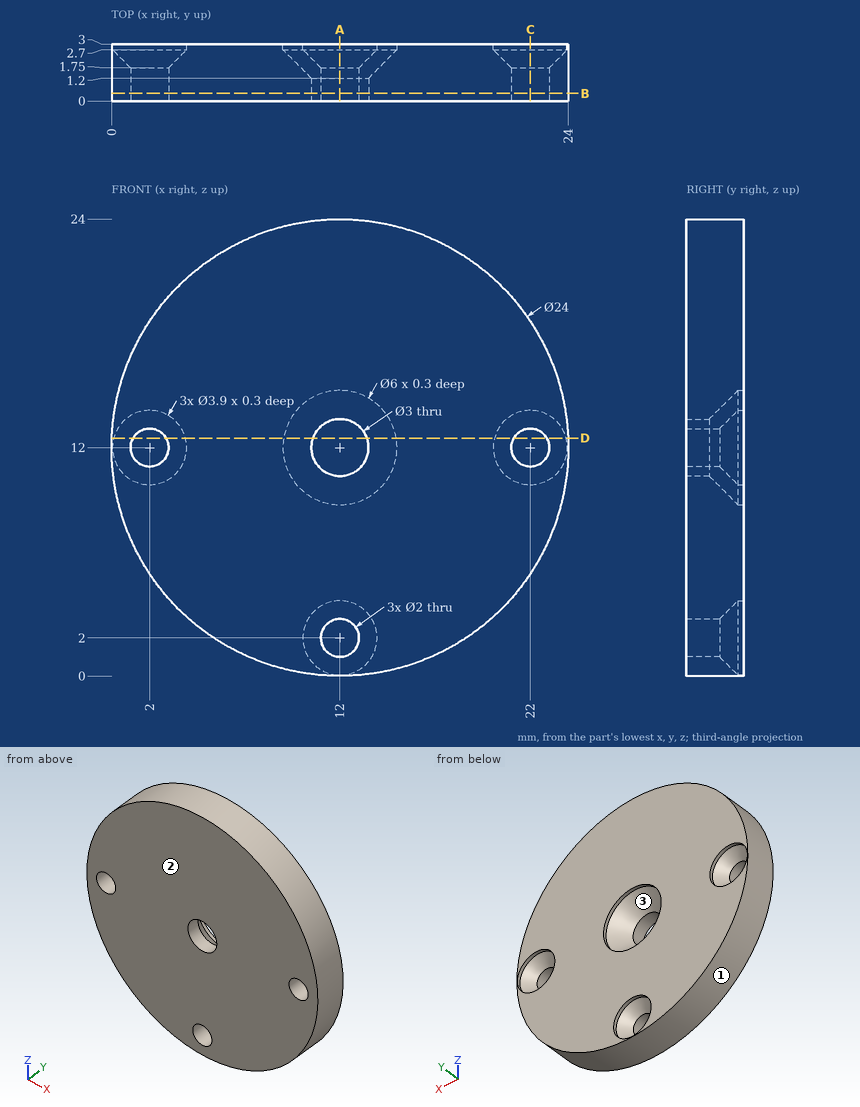
Part print with two shaded views. Sizes in mm from the minimum x, y, z corner. Coordinates: 2 decimals unless noted, no trailing zeros. Order: outer loops, then holes, each group sorted by start corner. A loop starts at its lowest first (then second) coordinate and runs counter-clockwise, first axis right, second up.
(1) Saw through at B-B, the plane y = 0.4. Write the cut outline in (x, z).
Solution:
outline: circle Ø24 at (12, 12); hole circle Ø2 at (2, 12); hole circle Ø3 at (12, 12); hole circle Ø2 at (12, 2); hole circle Ø2 at (22, 12)
(2) Saw through at C-C, the plane x = 22. Write the cut outline in (y, z), and give its area (3 significant figures).
Solution:
outline: (0, 5.37) - (3, 5.37) - (3, 10.05) - (2.7, 10.05) - (1.75, 11) - (0, 11) - close; (0, 13) - (1.75, 13) - (2.7, 13.95) - (3, 13.95) - (3, 18.63) - (0, 18.63) - close
area: 32.3 mm2
(3) Saw through at D-D, the plane z = 12.5. Count the separate pieces of the cut face and the enclosed holes in it, and give its area (3 significant figures).
Solution:
separate pieces: 4
enclosed holes: 0
area: 46.6 mm2
(4) Pin check, flat tips, straight feed: pin 1 Ø5 at (x, z) = (12, 12) entering from +Y; pin 2 Ø1 at (x, y) = (7, 2.5) entering from -Z; pin 3 Ø2.5 at (x, z) = (12, 2) entering from +Y. Stop position of each tip, or through.
Solution:
pin 1: stops at y = 2.2
pin 2: stops at z = 0.88
pin 3: stops at y = 2
(5) Drill centre lines: L1, parallel to Z at x = 12.5, y = 1.8; L2, parallel to Z at x = 11.5, y = 1.9; L3, parallel to X at y = 0.25, z = 12.5. Where is each one in solid material? Low to high.
Solution:
L1: z = 0.01 to 1.08, 2.92 to 9.96, 14.04 to 23.99
L2: z = 0.01 to 0.96, 3.04 to 9.86, 14.14 to 23.99
L3: x = 0.01 to 1.13, 2.87 to 10.59, 13.41 to 21.13, 22.87 to 23.99
(6) Mould opens along X. For the marked faces 1, 2 and 3 say: released by +X, released by -X, zero draft, split by the parting line, or undercut.
Solution:
face 1: split by the parting line
face 2: zero draft
face 3: undercut
(7) Saw through at A-A, the plane x = 12. Write the cut outline in (y, z), and give its area (3 significant figures).
Solution:
outline: (0, 0) - (3, 0) - (3, 0.05) - (2.7, 0.05) - (1.75, 1) - (0, 1) - close; (0, 3) - (1.75, 3) - (2.7, 3.95) - (3, 3.95) - (3, 9) - (2.7, 9) - (1.2, 10.5) - (0, 10.5) - close; (0, 13.5) - (1.2, 13.5) - (2.7, 15) - (3, 15) - (3, 24) - (0, 24) - close
area: 52.4 mm2
